```python
from build123d import *

# Parameters (mm, degrees)
SKETCH1_W           = 500
SKETCH1_H           = 570
BOSS_EXTRUDE1_DEPTH = 30
FILLET1_R           = 10
SKETCH3_W           = 500
SKETCH3_H           = 20
SKETCH3_W_2         = 24.124551532
SKETCH3_W_3         = 40.885345678
SKETCH3_W_4         = 75.086674906
CUT_EXTRUDE1_DEPTH  = 10


with BuildPart() as part:
    # Sketch1 → Boss-Extrude1 (new body)
    with BuildSketch(Plane.XY):
        with Locations((-250, -285)):
            Rectangle(SKETCH1_W, SKETCH1_H)
    extrude(amount=BOSS_EXTRUDE1_DEPTH)

    # Fillet1
    fillet1_edges = [part.edges().sort_by_distance(p)[0] for p in [
        (-500, -285, 30),
        (-250, -570, 30),
        (0, -285, 30),
        (-250, 0, 30),
    ]]
    fillet(fillet1_edges, radius=FILLET1_R)

    # Sketch3 → Cut-Extrude1 (cut)
    with BuildSketch(Plane.XY):
        with Locations((-250, -376.410467709)):
            Rectangle(SKETCH3_W, SKETCH3_H)
        with Locations((-512.062275766, -376.410467709)):
            Rectangle(SKETCH3_W_2, SKETCH3_H)
        with Locations((12.062275766, -376.410467709)):
            Rectangle(SKETCH3_W_2, SKETCH3_H)
        with Locations((20.442672839, -183.821390857)):
            Rectangle(SKETCH3_W_3, SKETCH3_H)
        with Locations((-250, -183.821390857)):
            Rectangle(SKETCH3_W, SKETCH3_H)
        with Locations((-537.543337453, -183.821390857)):
            Rectangle(SKETCH3_W_4, SKETCH3_H)
    extrude(amount=CUT_EXTRUDE1_DEPTH, mode=Mode.SUBTRACT)


solid = part.part
```
CAD build for the part. Positions are in the model's coordinates, mm. A direction names the side the tool comes from. Round coordinates to 2 decimals unless told otherwise and drop trailing zeros. Write each loop counter-clockwise with the first axis right and the second up, starting at its lowest first coordinate (ties: lowest second). Pieces come first, ordered by that corner, then holes. Notation, with made-up numbers: (75, 58) - (122, 58) arc R21 ccw to (122, 81) - close; hole circle Ø10 at (47, 16.25). An arc over 180 degrees is marked (long way). Write item = value, one per line. Start each with the question number.
Q1. Probe L1, parallel to Y at x = -60.5, z = 2.25; L2, parallel to Z at x = -316, y = -182; L3, parallel to Y at x = -162, z = 20.5. List the from-to ranges inside material, lowest first. Write a range as from..to.
Q2. Which spindle directions (+Z, -Z, +X, -X, +Y, -Y) get a long thin tool onto all of the face, cutting with end or side? Do faces 1 (the flat face through (-253, -86, 0)), 2 (the flat face through (-254, -184, 10)). Say none if no direction does.
Q3. Drop flat-ended pins along their axis: pin 1 (4 mm diameter, centred on x = -106, z = 26.5, fed in from -Y); pin 2 (1 mm diameter, centred on x = -220.5, z = 22.5, fed in from +Y); pin 3 (6 mm diameter, centred on x = -308, y = -185.5, fed in from -Z). Give the stop position or say it passes through.
Q4. Mould opens along Y. For faces 3 (the flat face through (-253, 0, 10)), 4 (the flat face through (-253, -376, 10)), 5 (the flat face through (-253, -570, 10)), 6 (the flat face through (-254, -279, 0)) say: pulls with the +Y half, pulls with the -Y half, needs draft (parallel to the pull), parting line crosses it, or undercut.
Q5. Band-saw the part on A-A (x = -306.5). Give the cut face in (y, z).
Answers below:
q1.L1 = -570..-386.41, -366.41..-193.82, -173.82..0
q1.L2 = 10..30
q1.L3 = -569.99..-0.01
q2.face_1 = -Z, +X, -X, +Y, -Y
q2.face_2 = -Z, +X, -X
q3.pin_1 = -568.93
q3.pin_2 = -0.2
q3.pin_3 = 10
q4.face_3 = pulls with the +Y half
q4.face_4 = undercut
q4.face_5 = pulls with the -Y half
q4.face_6 = needs draft
q5.outline = (-570, 0) - (-386.41, 0) - (-386.41, 10) - (-366.41, 10) - (-366.41, 0) - (-193.82, 0) - (-193.82, 10) - (-173.82, 10) - (-173.82, 0) - (0, 0) - (0, 20) arc R10 ccw to (-10, 30) - (-560, 30) arc R10 ccw to (-570, 20) - close
